Model file for the job. Use its own axes, mm. A direction names the side the tool comes from. Coordinates: 2 decimals unless noted, no trailing zeros. Write each loop counter-clockwise with the first axis right and the second up, starting at its lowest first coordinate (ties: lowest second). Pieces come first, ordered by that corner, then holes. Notation, with made-up numbers: (-20.5, -22.75) -> (27.5, -22.75) arc R26 cw to (27.5, 4.25) -> close; hole circle Ø7 at (51.25, -30.75). An arc over 180 degrees is marked (long way). Write item = value, one per line. Start each with the question number.
from build123d import *

# Parameters (mm, degrees)
BOSS_EXTRUDE1_DEPTH      = 0.75
BOSS_EXTRUDE1_DEPTH_BACK = 0.75
CUT_EXTRUDE1_DEPTH       = 188.923950642
LPATTERN1_COUNT          = 7
LPATTERN1_PITCH          = 50
MIRROR1_COPY_1_DEPTH     = 188.923950642
MIRROR1_COPY_2_DEPTH     = 188.923950642
MIRROR1_COPY_3_DEPTH     = 188.923950642
MIRROR1_COPY_4_DEPTH     = 188.923950642
MIRROR1_COPY_5_DEPTH     = 188.923950642
MIRROR1_COPY_6_DEPTH     = 188.923950642
SKETCH6_W                = 177.8
SKETCH6_H                = 254
SKETCH6_W_2              = 152.4
SKETCH6_H_2              = 228.6
BOSS_EXTRUDE2_DEPTH      = 11.5


with BuildPart() as part:
    # Sketch3 → Boss-Extrude1 (new, two sides: drawn at the far end of the back side and taken through both)
    with BuildSketch(Plane.XY.offset(-BOSS_EXTRUDE1_DEPTH_BACK)):
        Polygon((-105.41, 132.575), (-82.41, 155.575), (82.41, 155.575), (105.41, 132.575), (105.41, -132.575), (82.41, -155.575), (-82.41, -155.575), (-105.41, -132.575), align=None)
    extrude(amount=BOSS_EXTRUDE1_DEPTH + BOSS_EXTRUDE1_DEPTH_BACK)

    # Sketch4 → Cut-Extrude1 (cut, symmetric)
    with BuildSketch(Plane.XY):
        with BuildLine():
            Line((53, 149.225), (53, 155.575))
            Line((53, 155.575), (47, 155.575))
            Line((47, 155.575), (47, 149.225))
            ThreePointArc((47, 149.225), (50, 146.225), (53, 149.225))
        make_face()
    cut_extrude1 = extrude(amount=CUT_EXTRUDE1_DEPTH, both=True, mode=Mode.SUBTRACT)

    # LPattern1: Cut-Extrude1 ×7
    with Locations(*[(-i * LPATTERN1_PITCH, 0, 0) for i in range(1, LPATTERN1_COUNT)]):
        add(cut_extrude1, mode=Mode.SUBTRACT)

    # Mirror1: Cut-Extrude1 across plane
    add(cut_extrude1.mirror(Plane.ZX), mode=Mode.SUBTRACT)

    # Mirror1 copy 1 sketch → Mirror1 copy 1 (cut, symmetric)
    with BuildSketch(Plane(origin=(-50, 0, 0), x_dir=(1, 0, 0), z_dir=(0, 0, 1))):
        with BuildLine():
            Line((53, -149.225), (53, -155.575))
            Line((53, -155.575), (47, -155.575))
            Line((47, -155.575), (47, -149.225))
            ThreePointArc((47, -149.225), (50, -146.225), (53, -149.225))
        make_face()
    extrude(amount=MIRROR1_COPY_1_DEPTH, both=True, mode=Mode.SUBTRACT)

    # Mirror1 copy 2 sketch → Mirror1 copy 2 (cut, symmetric)
    with BuildSketch(Plane(origin=(-100, 0, 0), x_dir=(1, 0, 0), z_dir=(0, 0, 1))):
        with BuildLine():
            Line((53, -149.225), (53, -155.575))
            Line((53, -155.575), (47, -155.575))
            Line((47, -155.575), (47, -149.225))
            ThreePointArc((47, -149.225), (50, -146.225), (53, -149.225))
        make_face()
    extrude(amount=MIRROR1_COPY_2_DEPTH, both=True, mode=Mode.SUBTRACT)

    # Mirror1 copy 3 sketch → Mirror1 copy 3 (cut, symmetric)
    with BuildSketch(Plane(origin=(-150, 0, 0), x_dir=(1, 0, 0), z_dir=(0, 0, 1))):
        with BuildLine():
            Line((53, -149.225), (53, -155.575))
            Line((53, -155.575), (47, -155.575))
            Line((47, -155.575), (47, -149.225))
            ThreePointArc((47, -149.225), (50, -146.225), (53, -149.225))
        make_face()
    extrude(amount=MIRROR1_COPY_3_DEPTH, both=True, mode=Mode.SUBTRACT)

    # Mirror1 copy 4 sketch → Mirror1 copy 4 (cut, symmetric)
    with BuildSketch(Plane(origin=(-200, 0, 0), x_dir=(1, 0, 0), z_dir=(0, 0, 1))):
        with BuildLine():
            Line((53, -149.225), (53, -155.575))
            Line((53, -155.575), (47, -155.575))
            Line((47, -155.575), (47, -149.225))
            ThreePointArc((47, -149.225), (50, -146.225), (53, -149.225))
        make_face()
    extrude(amount=MIRROR1_COPY_4_DEPTH, both=True, mode=Mode.SUBTRACT)

    # Mirror1 copy 5 sketch → Mirror1 copy 5 (cut, symmetric)
    with BuildSketch(Plane(origin=(-250, 0, 0), x_dir=(1, 0, 0), z_dir=(0, 0, 1))):
        with BuildLine():
            Line((53, -149.225), (53, -155.575))
            Line((53, -155.575), (47, -155.575))
            Line((47, -155.575), (47, -149.225))
            ThreePointArc((47, -149.225), (50, -146.225), (53, -149.225))
        make_face()
    extrude(amount=MIRROR1_COPY_5_DEPTH, both=True, mode=Mode.SUBTRACT)

    # Mirror1 copy 6 sketch → Mirror1 copy 6 (cut, symmetric)
    with BuildSketch(Plane(origin=(-300, 0, 0), x_dir=(1, 0, 0), z_dir=(0, 0, 1))):
        with BuildLine():
            Line((53, -149.225), (53, -155.575))
            Line((53, -155.575), (47, -155.575))
            Line((47, -155.575), (47, -149.225))
            ThreePointArc((47, -149.225), (50, -146.225), (53, -149.225))
        make_face()
    extrude(amount=MIRROR1_COPY_6_DEPTH, both=True, mode=Mode.SUBTRACT)

    # Sketch6 → Boss-Extrude2 (add)
    with BuildSketch(Plane(origin=(0, 0, -0.75), x_dir=(-1, 0, 0), z_dir=(0, 0, -1))):
        Rectangle(SKETCH6_W, SKETCH6_H)
        Rectangle(SKETCH6_W_2, SKETCH6_H_2, mode=Mode.SUBTRACT)
    extrude(amount=-BOSS_EXTRUDE2_DEPTH)


solid = part.part
(1) Drill centre lines: line 1 along X through (y, z) = (90.5, 2.5); line 2 along Y through (x, z) = (-28, 9.5); line 3 along Y through (x, z) = (77.5, 8). Where is each one in solid material? Low to high.
(2) 3-axis set-ups, long thin cutter, end or side, ignore diameter. For faces 5 (the face through (1, 127, 6)), 6 (the face through (76.2, -2, 6)), 7 (the face through (-94.071, 143.914, -0.01)), 8 (the face through (1, -127, 6)), 9 (the face through (93.749, 144.236, -0.01)): which of +Z, -Z, +X, -X, +Y, -Y reach the whole face in a straight line?
(3) Saw through at A-A (z = 4.25). Give the cut face in (x, y), then the cut area to 3 significant figures.
(4) Saw through at C-C (y = 4). Give the cut face in (x, z).
(5) Mould opens along X. For faces 1 (the face through (-76.2, -2, 6)), 2 (the face through (1, -114.3, 6)), 3 (the face through (88.9, -2, 6)), 4 (the face through (-88.9, -2, 6)) say: released by +X, released by -X, zero draft, split by the parting line, or undercut.
(6) Saw through at B-B (x = -22.5). Give the cut face in (y, z) (3 decimals).
(7) Drop flat-ended pins along their axis: pin 1 Ø3 at (x, z) = (77, 8) entering from -Y; pin 2 Ø3 at (y, z) = (104, 4.5) entering from +X; pin 3 Ø1.2 at (y, z) = (153.5, 0) entering from +X (3 decimals); pin 4 Ø4 at (x, z) = (-46.5, 2) entering from +Y (3 decimals). Give the stop position or say it passes through.
Returned:
q1.line_1 = -88.9 to -76.2, 76.2 to 88.9
q1.line_2 = -127 to -114.3, 114.3 to 127
q1.line_3 = -127 to 127
q2.face_5 = +Z, +X, -X, +Y
q2.face_6 = +Z
q2.face_7 = +Z, -Z, -X, +Y
q2.face_8 = +Z, +X, -X, -Y
q2.face_9 = +Z, -Z, +X, +Y
q3.outline = (-88.9, -127) -> (88.9, -127) -> (88.9, 127) -> (-88.9, 127) -> close; hole (-76.2, -114.3) -> (76.2, -114.3) -> (76.2, 114.3) -> (-76.2, 114.3) -> close
q3.area = 10,300 mm2
q4.outline = (-105.41, -0.75) -> (105.41, -0.75) -> (105.41, 0.75) -> (88.9, 0.75) -> (88.9, 10.75) -> (76.2, 10.75) -> (76.2, 0.75) -> (-76.2, 0.75) -> (-76.2, 10.75) -> (-88.9, 10.75) -> (-88.9, 0.75) -> (-105.41, 0.75) -> close
q5.face_1 = undercut
q5.face_2 = undercut
q5.face_3 = released by +X
q5.face_4 = released by -X
q6.outline = (-155.575, -0.75) -> (155.575, -0.75) -> (155.575, 0.75) -> (127, 0.75) -> (127, 10.75) -> (114.3, 10.75) -> (114.3, 0.75) -> (-114.3, 0.75) -> (-114.3, 10.75) -> (-127, 10.75) -> (-127, 0.75) -> (-155.575, 0.75) -> close
q7.pin_1 = -127
q7.pin_2 = 88.9
q7.pin_3 = 85.085
q7.pin_4 = 155.575
